from build123d import *

# Parameters (mm, degrees)
CROQUIS1_R              = 4
CROQUIS1_R_2            = 1.75
SALIENTE_EXTRUIR1_DEPTH = 2.5
CROQUIS1_3_R            = 2.5
CROQUIS1_3_R_2          = 1.75
SALIENTE_EXTRUIR2_DEPTH = 11
REDONDEO1_R             = 2
REDONDEO2_R             = 2
CROQUIS2_R              = 3
CORTAR_EXTRUIR1_DEPTH   = 2
REDONDEO3_R             = 4


with BuildPart() as part:
    # Croquis1 → Saliente-Extruir1 (new, symmetric)
    with BuildSketch(Plane.XY):
        with BuildLine():
            Line((20.001432119, 0), (-20.001432119, 0))
            Line((-20.001432119, 0), (-14.963460754, -72.046347106))
            ThreePointArc((-14.963460754, -72.046347106), (0, -86), (14.963460754, -72.046347106))
            Line((14.963460754, -72.046347106), (20.001432119, 0))
        make_face()
        with Locations((0, -72.046347106)):
            Circle(CROQUIS1_R, mode=Mode.SUBTRACT)
        Polygon((12.515549555, -64.046347106), (-10.788577252, -64.046347106), (15.770666891, -17.496000466), align=None, mode=Mode.SUBTRACT)
        Polygon((-12.704099543, -61.349956664), (-16.011890152, -14.046347106), (14.28491785, -14.046347106), align=None, mode=Mode.SUBTRACT)
        with Locations((-15.5, -7.276347106)):
            Circle(CROQUIS1_R_2, mode=Mode.SUBTRACT)
        with Locations((15.5, -7.276347106)):
            Circle(CROQUIS1_R_2, mode=Mode.SUBTRACT)
    extrude(amount=SALIENTE_EXTRUIR1_DEPTH, both=True)

    # Croquis1_3 → Saliente-Extruir2 (add)
    # profile 1 of 2: a face of its own
    with BuildSketch(Plane.XY):
        with Locations((-15.5, -7.276347106)):
            Circle(CROQUIS1_3_R)
        with Locations((-15.5, -7.276347106)):
            Circle(CROQUIS1_3_R_2, mode=Mode.SUBTRACT)
    # profile 2 of 2: a face of its own
    with BuildSketch(Plane.XY):
        with Locations(Location((15.5, -7.276347106, 0), (0, 0, 180))):
            Circle(CROQUIS1_3_R)
        with Locations(Location((15.5, -7.276347106, 0), (0, 0, 180))):
            Circle(CROQUIS1_3_R_2, mode=Mode.SUBTRACT)
    extrude(amount=SALIENTE_EXTRUIR2_DEPTH)

    # Redondeo1
    redondeo1_edges = [part.edges().sort_by_distance(p)[0] for p in [
        (18, -7.276347106, 2.5),
        (-18, -7.276347106, 2.5),
    ]]
    fillet(redondeo1_edges, radius=REDONDEO1_R)

    # Redondeo2
    redondeo2_edges = [part.edges().sort_by_distance(p)[0] for p in [
        (-20.001432119, 0, 0),
        (20.001432119, 0, 0),
    ]]
    fillet(redondeo2_edges, radius=REDONDEO2_R)

    # Croquis2 → Cortar-Extruir1 (cut)
    with BuildSketch(Plane(origin=(0, 0, -2.5), x_dir=(-1, 0, 0), z_dir=(0, 0, -1))):
        with Locations((-15.5, -7.276347106)):
            Circle(CROQUIS2_R)
        with Locations((15.5, -7.276347106)):
            Circle(CROQUIS2_R)
    extrude(amount=-CORTAR_EXTRUIR1_DEPTH, mode=Mode.SUBTRACT)

    # Redondeo3
    redondeo3_edges = [part.edges().sort_by_distance(p)[0] for p in [
        (12.515549555, -64.046347106, 0),
        (15.770666891, -17.496000466, 0),
        (-10.788577252, -64.046347106, 0),
        (14.28491785, -14.046347106, 0),
        (-16.011890152, -14.046347106, 0),
        (-12.704099543, -61.349956664, 0),
    ]]
    fillet(redondeo3_edges, radius=REDONDEO3_R)


solid = part.part
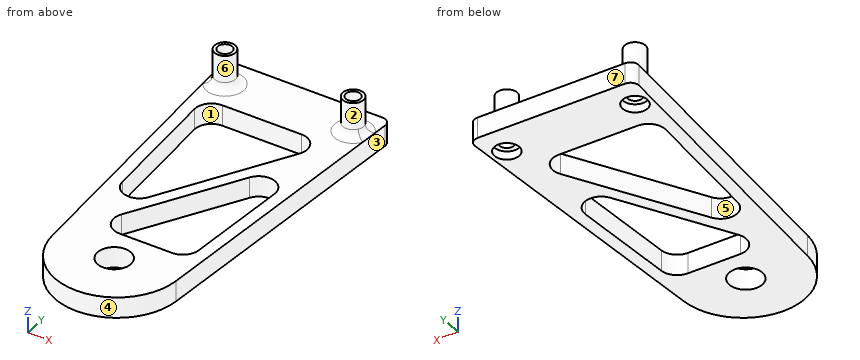
Can you work these out from the model? Positions are in its coordinate system, mm. Face numbers are marked on the shaded views. A direction names the side the tool comes from. Coordinates: 2 decimals unless noted, no trailing zeros. Write each loop counter-clockwise with the first axis right and the second up, starting at its lowest first coordinate (ties: lowest second). Pieces come first, ordered by that corner, then holes.
Q1. Please list where these lines run through material, in increasing order: L1, parallel to Y at x = -15.5, z = 6.75; L2, parallel to Y at x = 0, z = 0.65; L3, parallel to Y at x = -1, z = 1.5.
Results found:
L1: y = -9.78 to -9.03, -5.53 to -4.78
L2: y = -86 to -76.05, -68.05 to -64.05, -45.14 to -39.08, -14.05 to 0
L3: y = -85.97 to -75.92, -68.17 to -64.05, -46.89 to -40.84, -14.05 to 0
Q2. Which directions (+Z, -Z, +X, -X, +Y, -Y) give clear straight access to the entire face, cutting with the end or side of a thin tool? Please do the marked faces 1, 2 and 3.
Results found:
face 1: +Z, -Z
face 2: +Z
face 3: +Z, -Z, +X, -Y
Q3. Imagine slicing it at B-B, the plane y = -15.5. List the corners of the cut face in (x, z) for me, plus the area to 3 significant figures.
Results found:
outline: (-18.92, -2.5) - (-14.81, -2.5) - (-14.81, 2.5) - (-18.92, 2.5) - close; (10.48, -2.5) - (18.92, -2.5) - (18.92, 2.5) - (10.48, 2.5) - close
area: 62.7 mm2
Q4. Imagine slicing it at C-C, the plane z = 8. List the corners of the cut face in (x, y) for me, plus the area to 3 significant figures.
Results found:
outline: circle Ø5 at (-15.5, -7.28); circle Ø5 at (15.5, -7.28); hole circle Ø3.5 at (-15.5, -7.28); hole circle Ø3.5 at (15.5, -7.28)
area: 20.0 mm2
Q5. If we mould it in two halves opening along Y, with no side actions, what happens to the marked faces 4, 5, 6 and 7? For each: +Y half, -Y half, draft (parallel to the pull), parting line (faces both ways), or undercut.
Results found:
face 4: -Y half
face 5: undercut
face 6: parting line
face 7: +Y half
Q6. Imagine slicing it at A-A, the plane x = 0. List the corners of the cut face in (y, z) for me.
Results found:
outline: (-86, -2.5) - (-76.05, -2.5) - (-76.05, 2.5) - (-86, 2.5) - close; (-68.05, -2.5) - (-64.05, -2.5) - (-64.05, 2.5) - (-68.05, 2.5) - close; (-45.14, -2.5) - (-39.08, -2.5) - (-39.08, 2.5) - (-45.14, 2.5) - close; (-14.05, -2.5) - (0, -2.5) - (0, 2.5) - (-14.05, 2.5) - close
Q7. Imagine slicing it at D-D, the plane y = -71. List the corners of the cut face in (x, z) for me.
Results found:
outline: (-15.04, -2.5) - (-3.86, -2.5) - (-3.86, 2.5) - (-15.04, 2.5) - close; (3.86, -2.5) - (15.04, -2.5) - (15.04, 2.5) - (3.86, 2.5) - close
Q8. For P1, Ø6, axis at x = 15.5, z = 9, coming from the -Y side; P2, Ø8, axis at x = -7.5, y = -59, coming from the +Z side; P3, Ø7, axis at x = 0, y = -72.05, coming from the -Z side (3 decimals); P4, Ø1, axis at y = -11.5, z = 1.5, coming from the +X side, each with a flat end and sliding along its axis, tell me the tip position at first contact or that it passes through.
Results found:
P1: stops at y = -9.78
P2: stops at z = 2.5
P3: passes through
P4: stops at x = 19.23
